Geometry check sheet. Reference: the model listing, model coordinates, mm. Give positions to 0.01 mm unless a question says otherwise; leave off trailing zeros. Order: outer loops, then holes, each group sorted by start corner. A loop starts at its lowest first (then second) coordinate and runs counter-clockwise, first axis right, second up.
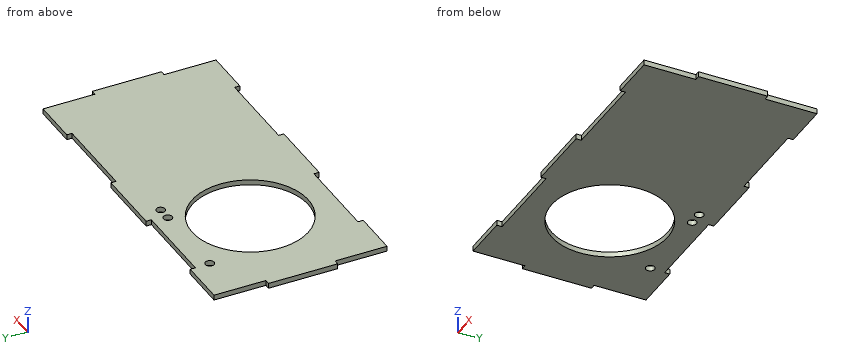
```python
from build123d import *

# Parameters (mm, degrees)
ESQUISSE2_R             = 33.5
BOSS_EXTRU_1_DEPTH      = 3
ENL_V_MAT_EXTRU_1_REACH = 174.782
ESQUISSE3_R             = 2.55


with BuildPart() as part:
    # Esquisse2 → Boss.-Extru.1 (new body)
    with BuildSketch(Plane.XY):
        Polygon((26.963895135, 9.191113465), (66.963895135, 9.191113465), (66.963895135, 6.191113465), (116.963895135, 6.191113465), (116.963895135, 9.191113465), (143.963895135, 9.191113465), (143.963895135, -20.808886535), (146.963895135, -20.808886535), (146.963895135, -60.808886535), (143.963895135, -60.808886535), (143.963895135, -90.808886535), (116.963895135, -90.808886535), (116.963895135, -87.808886535), (66.963895135, -87.808886535), (66.963895135, -90.808886535), (26.963895135, -90.808886535), (26.963895135, -87.808886535), (-23.036104865, -87.808886535), (-23.036104865, -90.808886535), (-50.036104865, -90.808886535), (-50.036104865, -60.808886535), (-53.036104865, -60.808886535), (-53.036104865, -20.808886535), (-50.036104865, -20.808886535), (-50.036104865, 9.191113465), (-23.036104865, 9.191113465), (-23.036104865, 6.191113465), (26.963895135, 6.191113465), align=None)
        with Locations((6.963895135, -40.808886535)):
            Circle(ESQUISSE2_R, mode=Mode.SUBTRACT)
    extrude(amount=BOSS_EXTRU_1_DEPTH)

    # Esquisse3 → Enlèv. mat.-Extru.1 (cut, up to next)
    with BuildSketch(Plane.XY.offset(3), mode=Mode.PRIVATE) as enl_v_mat_extru_1_sk1:
        with Locations((24.835002906, -2.259814335)):
            Circle(ESQUISSE3_R)
    enl_v_mat_extru_1_tool1 = extrude(enl_v_mat_extru_1_sk1.sketch, amount=-ENL_V_MAT_EXTRU_1_REACH, mode=Mode.PRIVATE) & part.part
    # Esquisse3 → Enlèv. mat.-Extru.1 (cut, up to next)
    with BuildSketch(Plane.XY.offset(3), mode=Mode.PRIVATE) as enl_v_mat_extru_1_sk2:
        with Locations((32.903794199, -2.259814335)):
            Circle(ESQUISSE3_R)
    enl_v_mat_extru_1_tool2 = extrude(enl_v_mat_extru_1_sk2.sketch, amount=-ENL_V_MAT_EXTRU_1_REACH, mode=Mode.PRIVATE) & part.part
    # Esquisse3 → Enlèv. mat.-Extru.1 (cut, up to next)
    with BuildSketch(Plane.XY.offset(3), mode=Mode.PRIVATE) as enl_v_mat_extru_1_sk3:
        with Locations((-22.713231498, -2.259814335)):
            Circle(ESQUISSE3_R)
    enl_v_mat_extru_1_tool3 = extrude(enl_v_mat_extru_1_sk3.sketch, amount=-ENL_V_MAT_EXTRU_1_REACH, mode=Mode.PRIVATE) & part.part
    add(enl_v_mat_extru_1_tool1.solids().sort_by_distance((24.835003, -2.259814, 3))[0], mode=Mode.SUBTRACT)
    add(enl_v_mat_extru_1_tool2.solids().sort_by_distance((32.903794, -2.259814, 3))[0], mode=Mode.SUBTRACT)
    add(enl_v_mat_extru_1_tool3.solids().sort_by_distance((-22.713231, -2.259814, 3))[0], mode=Mode.SUBTRACT)


solid = part.part
```
Q1. Gauge pin test, flat ends, axial feed: P1, Ø0.9, axis at x = 5, z = 1.5, coming from the +Y side; P2, Ø1.5, axis at y = 8, z = 1.5, coming from the +X side; P3, Ø1.5, axis at x = 146, z = 1.5, coming from the -Y side. Record the tip position at first contact, or that the pin passes through.
Q2. Cross-section at B-B, the plane x = 11. Record the boundary of the cut face in (y, z).
Q3. Cross-section at D-D, the plane x = 99. Record the boundary of the cut face in (y, z), and give its area (3 significant figures).
Q4. Cross-section at A-A, the plane y = -37.5. Record the boundary of the cut face in (x, z).
Q5. Thickness scan on L1, parallel to X at y = -1, z = 2.25; L2, parallel to Y at x = 75.5, z = 0.55; L3, parallel to X at y = -39.5, z = 2.55. Record the ranges inside material, lowest first.
Q6. Cross-section at C-C, the plane z = 2.2. Give the number of separate pieces and of enclosed holes in the cut face, and give its area (3 significant figures).
Answers follow:
1. P1: stops at y = 6.19
1. P2: stops at x = 143.96
1. P3: stops at y = -60.81
2. outline: (-87.81, 0) - (-74.06, 0) - (-74.06, 3) - (-87.81, 3) - close; (-7.55, 0) - (6.19, 0) - (6.19, 3) - (-7.55, 3) - close
3. outline: (-87.81, 0) - (6.19, 0) - (6.19, 3) - (-87.81, 3) - close
3. area: 282 mm2
4. outline: (-53.04, 0) - (-26.37, 0) - (-26.37, 3) - (-53.04, 3) - close; (40.3, 0) - (146.96, 0) - (146.96, 3) - (40.3, 3) - close
5. L1: x = -50.04 to -24.93, -20.5 to 22.62, 27.05 to 30.69, 35.12 to 143.96
5. L2: y = -87.81 to 6.19
5. L3: x = -53.04 to -26.51, 40.44 to 146.96
6. separate pieces: 1
6. enclosed holes: 4
6. area: 15,500 mm2
